Check sheet for the modelled part. Datum: model origin and axes. Units: mm. Face numbers are marked on the shaded views. A direction names the side the tool comes from. Round coordinates to 2 decimals unless told otherwise and drop trailing zeros. Loops run counter-clockwise (first coordinate to the right, second up) from the corner with the lowest first, then second, coordinate; pieces in that order, holes last. Notation, with made-up numbers: (-7, -35.5) -> (19, -35.5) arc R17 ccw to (19, -25.5) -> close; hole circle Ø3 at (-23.5, -22.5). An arc over 180 degrees is marked (long way). Use one line per item in the form item = value. Start each with the question number.
(1) Material ranges on probe 1 along Y at (x, z) = (9.5, 21); probe 2 along X at (y, z) = (-31.5, 16); probe 3 along X at (y, z) = (-22.5, 4), recorded low to high. Write a range as [from, to].
(2) Sectioned sample at B-B (x = -3). Record the cut outline in (y, z), and give its area (3 significant figures).
(3) Go/stop test with flat-tipped pins: pin 1 (3 mm diameter, centred on x = 1.5, z = 24, fed in from +Y); pin 2 (2 mm diameter, centred on x = 14.5, z = 26, fed in from -Y); pin 3 (6 mm diameter, centred on y = -21, z = 3.5, fed in from +X); pin 4 (2 mm diameter, centred on y = -26, z = 6, fed in from +X). Record where each tip stops, or that it passes through.
(4) Set-up check for the marked faces 1, 2 and 3: record each of +Z, -Z, +X, -X, +Y, -Y from which the full face is reachable in a straight line by a thin tool's end or side.
(5) Sectioned sample at D-D (z = 4). Record the cut outline in (x, y).
(6) Sectioned sample at C-C (y = -5.5). Record the cut outline in (x, z).
(7) Sectioned sample at A-A (z = 18). Record the cut outline in (x, y), and give its area (3 significant figures).
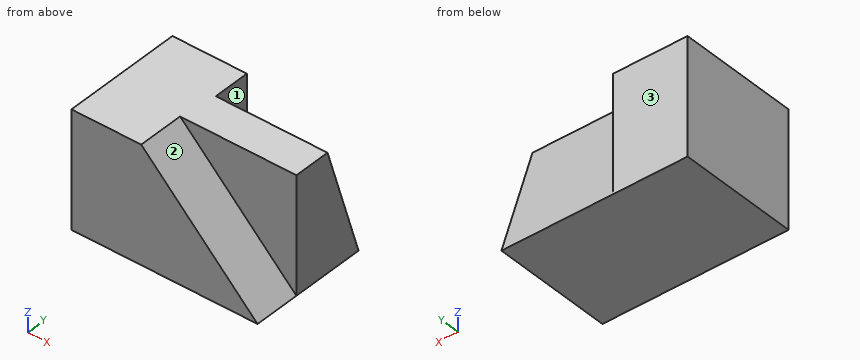
from build123d import *

# Parameters (mm, degrees)
F1_DEPTH = 33.02
F3_DEPTH = 12.7
F5_DEPTH = 30.48


with BuildPart() as f1:
    # F0 (on Front) → F1 (new body)
    with BuildSketch(Plane.XZ):
        Polygon((-25.4, 0), (0, 0), (25.4, 0), (25.4, 31.75), (-25.4, 31.75), align=None)
    extrude(amount=F1_DEPTH)

    # F2 (on face) → F3 (cut)
    with BuildSketch(Plane.XZ.offset(33.02)):
        Polygon((25.4, 31.75), (-6.357383, 31.75), (25.4, 0), align=None)
    extrude(amount=-F3_DEPTH, mode=Mode.SUBTRACT)

    # F4 (on face) → F5 (cut)
    with BuildSketch(Plane.YZ.offset(25.4)):
        Polygon((-10.16, 31.75), (0, 0), (0, 31.75), align=None)
    extrude(amount=-F5_DEPTH, mode=Mode.SUBTRACT)


solid = f1.part
Checks:
q1.probe_1 = [-20.32, -6.72]
q1.probe_2 = [-25.4, 9.4]
q1.probe_3 = [-25.4, 21.4]
q2.outline = (-33.02, 0) -> (0, 0) -> (-10.16, 31.75) -> (-20.32, 31.75) -> (-20.32, 28.39) -> (-33.02, 28.39) -> close
q2.area = 844 mm2
q3.pin_1 = -7.2
q3.pin_2 = -20.32
q3.pin_3 = 25.4
q3.pin_4 = 20.4
q4.face_1 = +Z, +X, +Y
q4.face_2 = +Z, +X, -Y
q4.face_3 = +Z, -Z, +X, -X, +Y
q5.outline = (-25.4, -33.02) -> (21.4, -33.02) -> (21.4, -20.32) -> (25.4, -20.32) -> (25.4, -1.28) -> (-5.08, -1.28) -> (-5.08, 0) -> (-25.4, 0) -> close
q6.outline = (-25.4, 0) -> (25.4, 0) -> (25.4, 17.19) -> (-5.08, 17.19) -> (-5.08, 31.75) -> (-25.4, 31.75) -> close
q7.outline = (-25.4, -33.02) -> (7.4, -33.02) -> (7.4, -20.32) -> (25.4, -20.32) -> (25.4, -5.76) -> (-5.08, -5.76) -> (-5.08, 0) -> (-25.4, 0) -> close
q7.area = 1,270 mm2
